Here's how the part is built. I have some questions about the finished solid (model axes, mm). Coordinates: 2 decimals unless noted, no trailing zeros. Loops run counter-clockwise (first coordinate to the right, second up) from the corner with the lowest first, then second, coordinate; pieces in that order, holes last.
```python
from build123d import *

# Parameters (mm, degrees)
SKETCH1_R           = 1.5
BOSS_EXTRUDE1_DEPTH = 6
SKETCH2_R           = 1.5
BOSS_EXTRUDE2_DEPTH = 4
SKETCH3_R           = 1.5
CUT_EXTRUDE1_DEPTH  = 10


with BuildPart() as part:
    # Sketch1 → Boss-Extrude1 (new body)
    with BuildSketch(Plane(origin=(0, 0, 0), x_dir=(1, 0, 0), z_dir=(0, 1, 0))):
        with BuildLine():
            Line((0, 8), (122, 8))
            ThreePointArc((122, 8), (130, 0), (122, -8))
            Line((122, -8), (0, -8))
            ThreePointArc((0, -8), (-8, 0), (0, 8))
        make_face()
        Circle(SKETCH1_R, mode=Mode.SUBTRACT)
        with Locations((122, 0)):
            Circle(SKETCH1_R, mode=Mode.SUBTRACT)
    extrude(amount=BOSS_EXTRUDE1_DEPTH)

    # Sketch2 → Boss-Extrude2 (add)
    with BuildSketch(Plane(origin=(0, 6, 0), x_dir=(1, 0, 0), z_dir=(0, 1, 0))):
        with BuildLine():
            Line((4, 8), (4, 15))
            ThreePointArc((4, 15), (0, 19), (-4, 15))
            Line((-4, 15), (-4, 6.92820323))
            ThreePointArc((-4, 6.92820323), (-2.070552361, 7.72740661), (0, 8))
            Line((0, 8), (4, 8))
        make_face()
        with Locations((0, 15)):
            Circle(SKETCH2_R, mode=Mode.SUBTRACT)
        with BuildLine():
            Line((4, -15), (4, -8))
            Line((4, -8), (0, -8))
            ThreePointArc((0, -8), (-2.070552361, -7.72740661), (-4, -6.92820323))
            Line((-4, -6.92820323), (-4, -15))
            ThreePointArc((-4, -15), (0, -19), (4, -15))
        make_face()
        with Locations((0, -15)):
            Circle(SKETCH2_R, mode=Mode.SUBTRACT)
        with BuildLine():
            Line((118, 15), (118, 8))
            Line((118, 8), (122, 8))
            ThreePointArc((122, 8), (124.070552361, 7.72740661), (126, 6.92820323))
            Line((126, 6.92820323), (126, 15))
            ThreePointArc((126, 15), (122, 19), (118, 15))
        make_face()
        with Locations((122, 15)):
            Circle(SKETCH2_R, mode=Mode.SUBTRACT)
        with BuildLine():
            Line((122, -8), (118, -8))
            Line((118, -8), (118, -15))
            ThreePointArc((118, -15), (122, -19), (126, -15))
            Line((126, -15), (126, -6.92820323))
            ThreePointArc((126, -6.92820323), (124.070552361, -7.72740661), (122, -8))
        make_face()
        with Locations((122, -15)):
            Circle(SKETCH2_R, mode=Mode.SUBTRACT)
    extrude(amount=-BOSS_EXTRUDE2_DEPTH)

    # Sketch3 → Cut-Extrude1 (cut)
    with BuildSketch(Plane(origin=(0, 6, 0), x_dir=(1, 0, 0), z_dir=(0, 1, 0))):
        with Locations((61, 0)):
            Circle(SKETCH3_R)
    extrude(amount=-CUT_EXTRUDE1_DEPTH, mode=Mode.SUBTRACT)


solid = part.part
```
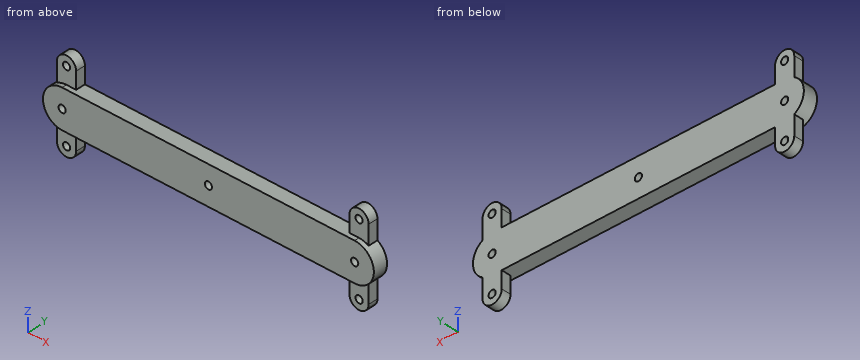
1. For pin 1 (2.5 mm diameter, centred on x = 120, z = -13, fed in from -Y); pin 2 (1.5 mm diameter, centred on x = 83, z = 9.5, fed in from +Y); pin 3 (4 mm diameter, centred on x = 122, z = 15, fed in from +Y); pin 4 (1.2 mm diameter, centred on y = 3.5, z = -9, fed in from +X), each with a flat end and sliding along its axis, tell me the tip position at first contact or that it passes through.
2. I want a section at C-C (x = 61). Please give me the cut outline in (y, z), then the cut area to 3 significant figures.
3. I need wall thicknesses on line 1 along Z through (x, y) = (0, 2.05); line 2 along X through (y, z) = (4.7, 0); line 3 along X through (y, z) = (3, -15). Which ranges of each line are inside material? Lowest first, please.
4. I want a section at A-A (y = 1.1). Please give me the cut outline in (x, z), then the cut area to 3 significant figures.
5. I want a section at D-D (z = 0). Please give me the cut outline in (x, y).
6. I want a section at B-B (z = 11). Please give me the cut outline in (x, y), then the cut area to 3 significant figures.
Response values:
1. pin 1: stops at y = 2
1. pin 2: passes through
1. pin 3: stops at y = 6
1. pin 4: stops at x = 126
2. outline: (0, -8) - (6, -8) - (6, -1.5) - (0, -1.5) - close; (0, 1.5) - (6, 1.5) - (6, 8) - (0, 8) - close
2. area: 78.0 mm2
3. line 1: z = -19 to -16.5, -13.5 to -1.5, 1.5 to 13.5, 16.5 to 19
3. line 2: x = -8 to -1.5, 1.5 to 59.5, 62.5 to 120.5, 123.5 to 130
3. line 3: x = -4 to -1.5, 1.5 to 4, 118 to 120.5, 123.5 to 126
4. outline: (0, -8) - (122, -8) arc R8 ccw to (122, 8) - (0, 8) arc R8 ccw to start; hole circle Ø3 at (0, 0); hole circle Ø3 at (61, 0); hole circle Ø3 at (122, 0)
4. area: 2,130 mm2
5. outline: (-8, 0) - (-1.5, 0) - (-1.5, 6) - (-8, 6) - close; (1.5, 0) - (59.5, 0) - (59.5, 6) - (1.5, 6) - close; (62.5, 0) - (120.5, 0) - (120.5, 6) - (62.5, 6) - close; (123.5, 0) - (130, 0) - (130, 6) - (123.5, 6) - close
6. outline: (-4, 2) - (4, 2) - (4, 6) - (-4, 6) - close; (118, 2) - (126, 2) - (126, 6) - (118, 6) - close
6. area: 64.0 mm2
